Work out the finished part from the listing and answer in its coordinate system (mm). A direction names the side the tool comes from. Give positions to 0.01 mm unless a question says otherwise; leave off trailing zeros. Order: outer loops, then holes, each group sorted by start corner. A loop starts at its lowest first (then second) coordinate and runs counter-clockwise, first axis right, second up. Notation, with made-up numbers: (-5, 43.5) - (28, 43.5) arc R21 ccw to (28, 71.5) - close; hole circle Ø9 at (-34, 18.5). An arc over 180 degrees is marked (long way). Put each result on its own line as item: value.
Autodesk Inventor part; units mm, degrees
ref_plane "YZ Plane" through (0, 0, 0) normal (1, 0, 0) x (0, 1, 0)
ref_plane "XZ Plane" through (0, 0, 0) normal (0, 1, 0) x (-1, 0, 0)
ref_plane "XY Plane" through (0, 0, 0) normal (0, 0, 1) x (1, 0, 0)
sketch "Sketch1" plane through (0, 0, 0) normal (0, 0, 1) x (1, 0, 0)
  line L0 (0, 0) -> (0, 70) construction
  circle A0 centre (0, 0) radius 2.5
  circle A1 centre (0, 70) radius 2.5
  line L1 (0, 0) -> (125, 0) construction
  circle A2 centre (125, 0) radius 2.5
  circle A3 centre (125, 70) radius 2.5
  line L2 (-8.5, -16) -> (133.5, -16)
  line L3 (133.5, -16) -> (133.5, 86)
  line L4 (133.5, 86) -> (-8.5, 86)
  line L5 (-8.5, 86) -> (-8.5, -16)
  point P0 (62.5, 0)
  point P1 (62.5, -16)
  point P2 (0, 35)
  point P3 (-8.5, 35)
  dimension "d0" = 70
  dimension "d1" = 5
  dimension "d2" = 5
  dimension "d3" = 5
  dimension "d4" = 5
  dimension "d5" = 125
  dimension "d6" = 142
  dimension "d7" = 102
extrude "Extrusion1" add sketch "Sketch1" along normal blind 5
sketch "Sketch2" plane through (0, 0, 5) normal (0, 0, 1) x (1, 0, 0)
  line L0 (6.5, 60) -> (118.5, 60)
  line L1 (118.5, 60) -> (118.5, 10)
  line L2 (118.5, 10) -> (6.5, 10)
  line L3 (6.5, 10) -> (6.5, 60)
  line L4 (-8.5, 86) -> (-8.5, -16)
  line L5 (133.5, 86) -> (-8.5, 86)
  point P0 (0, 0)
  point P1 (62.5, 60)
  point P2 (62.5, 86)
  point P3 (6.5, 35)
  point P4 (-8.5, 35)
  dimension "d10" = 15
  dimension "d11" = 50
extrude "Extrusion2" cut sketch "Sketch2" against normal through all
sketch "Sketch3" plane through (-8.5, 86, 0) normal (0, 1, 0) x (1, 0, 0)
  line L0 (142, 0) -> (142, -5)
  line L1 (142, -5) -> (0, -5)
  line L2 (0, -5) -> (0, 80)
  line L3 (0, 80) -> (142, 80)
  line L4 (142, 80) -> (142, -5)
  point P0 (8.5, 0)
  dimension "d17" = 85
extrude "Extrusion3" add sketch "Sketch3" along normal blind 2
sketch "Sketch4" plane through (-8.5, -16, 0) normal (0, -1, 0) x (1, 0, 0)
  line L0 (142, 0) -> (0, 0)
  line L1 (0, 0) -> (0, -80)
  line L2 (0, -80) -> (142, -80)
  line L3 (142, -80) -> (142, 0)
  line L4 (0, 0) -> (142, 0)
  line L5 (142, 0) -> (142, 5)
  line L6 (0, 5) -> (142, 5)
  line L7 (0, 0) -> (0, 5)
  point P0 (8.5, 0)
extrude "Extrusion4" add sketch "Sketch4" along normal blind 2
sketch "Sketch5" plane through (-8.5, 86, -80) normal (-1, 0, 0) x (0, 0, 1)
  line L0 (85, -104) -> (85, 2)
  line L1 (0, -102) -> (0, -104)
  line L2 (85, 2) -> (0, 2)
  line L3 (0, 2) -> (0, -104)
  line L4 (0, -104) -> (85, -104)
  line L5 (85, -104) -> (85, 2)
  point P0 (80, -86)
extrude "Extrusion5" add sketch "Sketch5" along normal blind 2
sketch "Sketch6" plane through (133.5, 86, 0) normal (1, 0, 0) x (0, 0, -1)
  line L0 (-5, -104) -> (-5, 2)
  line L1 (-5, -104) -> (80, -104)
  line L2 (80, -104) -> (80, 2)
  line L3 (80, 2) -> (-5, 2)
  line L4 (-5, 2) -> (-5, -104)
  point P0 (0, -86)
extrude "Extrusion6" add sketch "Sketch6" along normal blind 2
sketch "Sketch7" plane through (0, 0, 5) normal (0, 0, 1) x (1, 0, 0)
  line L0 (118.5, 10) -> (6.5, 10) construction
  line L1 (6.5, 60) -> (118.5, 60) construction
  line L2 (6.5, 10) -> (6.5, 60) construction
  line L3 (118.5, 60) -> (118.5, 10) construction
  line L4 (6.5, 60) -> (61.5, 60)
  line L5 (61.5, 60) -> (61.5, 50)
  line L6 (61.5, 50) -> (6.5, 50)
  line L7 (6.5, 50) -> (6.5, 60)
  line L8 (118.5, 10) -> (63.5, 10)
  line L9 (63.5, 10) -> (63.5, 20)
  line L10 (63.5, 20) -> (118.5, 20)
  line L11 (118.5, 20) -> (118.5, 10)
  line L12 (118.5, 10) -> (6.5, 10)
  line L13 (6.5, 60) -> (118.5, 60)
  line L14 (6.5, 10) -> (6.5, 60)
  point P0 (0, 0)
  point P1 (62.5, 10)
  point P2 (62.5, 60)
  point P3 (6.5, 35)
  dimension "d26" = 55
  dimension "d27" = 10
  dimension "d28" = 55
  dimension "d29" = 10
extrude "Extrusion7" add sketch "Sketch7" against normal blind 5
chamfer "Chamfer2" distance 3 angle 45 4 edges at (35, 10, 0) (90, 60, 0) (91, 20, 5) (34, 50, 5)
sketch "Sketch8" plane through (135.5, 86, 0) normal (1, 0, 0) x (0, 0, -1)
  line L0 (80, -104) -> (80, 2)
  line L1 (80, -102) -> (80, 0)
  line L2 (80, -51) -> (93.9386, -51)
  line L3 (80, -78.0836) -> (55, -78.0836)
  line L4 (55, -78.0836) -> (55, -58.0836)
  line L5 (55, -58.0836) -> (80, -58.0836)
  line L6 (80, -58.0836) -> (80, -78.0836)
  point P0 (0, -86)
  dimension "d36" = 20
  dimension "d37" = 25
  dimension "d40" = 7.0836
extrude "Extrusion8" cut sketch "Sketch8" against normal blind 10
sketch "Sketch9" plane through (-10.5, 86, -80) normal (-1, 0, 0) x (0, 0, 1)
  line L0 (0, -58.0836) -> (0, 0)
  line L1 (0, -31) -> (25, -31)
  line L2 (25, -31) -> (25, -71)
  line L3 (25, -71) -> (0, -71)
  line L4 (0, -71) -> (0, -31)
  line L5 (0, 2) -> (0, -104)
  line L6 (0, -71) -> (25, -71)
  line L7 (25, -71) -> (25, -31)
  line L8 (25, -31) -> (0, -31)
  line L9 (0, -31) -> (0, -71)
  point P0 (80, -86)
  point P1 (0, -51)
  dimension "d41" = 40
  dimension "d42" = 25
extrude "Extrusion9" cut sketch "Sketch9" against normal blind 10
sketch "Sketch10" plane through (-10.5, 86, -80) normal (-1, 0, 0) x (0, 0, 1)
  circle A0 centre (12.5, -93) radius 1.5
  circle A1 centre (12.5, -9) radius 1.5
  line L0 (12.5, -93) -> (12.5, -9) construction
  line L1 (85, -104) -> (85, 2)
  line L2 (25, -71) -> (0, -71)
  point P0 (80, -86)
  point P1 (85, -51)
  point P2 (12.5, -51)
  point P3 (12.5, -71)
  point P4 (12.5, -71)
  dimension "d45" = 3
  dimension "d46" = 3
  dimension "d47" = 84
extrude "Extrusion10" cut sketch "Sketch10" against normal blind 10
sketch "Sketch11" plane through (0, 0, 5) normal (0, 0, 1) x (1, 0, 0)
  circle A0 centre (0, 0) radius 2.5
  circle A1 centre (0, 70) radius 2.5
  circle A2 centre (125, 0) radius 2.5
  circle A3 centre (125, 70) radius 2.5
extrude "Extrusion11" add sketch "Sketch11" against normal blind 5
sketch "Sketch12" plane through (0, 0, 5) normal (0, 0, 1) x (1, 0, 0)
  line L0 (118.5, 20) -> (118.5, 63)
  line L1 (6.5, 7) -> (118.5, 7)
  line L2 (118.5, 7) -> (118.5, 63)
  line L3 (118.5, 63) -> (6.5, 63)
  line L4 (6.5, 63) -> (6.5, 7)
  point P0 (0, 0)
extrude "Extrusion12" cut sketch "Sketch12" along normal through all both and the other way through all
sketch "Sketch13" plane through (135.5, 86, 0) normal (1, 0, 0) x (0, 0, -1)
  line L0 (55, -58.0836) -> (80, -58.0836)
  line L1 (55, -78.0836) -> (55, -58.0836)
  line L2 (80, -78.0836) -> (55, -78.0836)
  line L3 (80, -58.0836) -> (80, -78.0836)
  line L4 (80, -71) -> (80, -102)
  point P0 (0, -86)
extrude "Extrusion13" add sketch "Sketch13" against normal blind 2
sketch "Sketch15" plane through (135.5, 86, 0) normal (1, 0, 0) x (0, 0, -1)
  line L0 (50, -31) -> (70, -31)
  line L1 (70, -31) -> (70, -16)
  line L2 (70, -16) -> (50, -16)
  line L3 (50, -16) -> (50, -31)
  line L4 (80, -104) -> (80, 2)
  line L5 (80, 2) -> (-5, 2)
  point P0 (0, -86)
  dimension "d64" = 20
  dimension "d65" = 15
  dimension "d66" = 10
  dimension "d67" = 18
extrude "Extrusion15" cut sketch "Sketch15" against normal blind 10
sketch "Sketch16" plane through (135.5, 86, 0) normal (1, 0, 0) x (0, 0, -1)
  line L0 (70, -31) -> (50, -31) construction
  line L1 (50, -16) -> (70, -16) construction
  line L2 (50, -31) -> (50, -16) construction
  line L3 (70, -16) -> (70, -31) construction
  line L4 (70, -31) -> (70, -16) construction
  line L5 (70, -31) -> (38, -31) construction
  line L6 (38, -31) -> (38, -71) construction
  line L7 (38, -71) -> (80, -71) construction
  line L8 (80, -71) -> (80, -31) construction
  line L9 (43, -66) -> (43, -36) construction
  line L10 (43, -36) -> (75, -36) construction
  line L11 (75, -36) -> (75, -66) construction
  line L12 (75, -66) -> (43, -66) construction
  line L13 (43, -36) -> (75, -36)
  line L14 (75, -36) -> (75, -38)
  line L15 (75, -38) -> (43, -38)
  line L16 (43, -38) -> (43, -36)
  line L17 (75, -66) -> (43, -66)
  line L18 (43, -66) -> (43, -64)
  line L19 (43, -64) -> (75, -64)
  line L20 (75, -64) -> (75, -66)
  line L21 (75, -45) -> (43, -45)
  line L22 (43, -43) -> (75, -43) construction
  line L23 (43, -43) -> (75, -43)
  line L24 (75, -43) -> (75, -45)
  line L25 (43, -45) -> (43, -43)
  line L26 (75, -43) -> (75, -73) construction
  line L27 (75, -52) -> (43, -52)
  line L28 (43, -50) -> (75, -50) construction
  line L29 (43, -50) -> (75, -50)
  line L30 (75, -50) -> (75, -52)
  line L31 (43, -52) -> (43, -50)
  line L32 (75, -50) -> (75, -80) construction
  line L33 (75, -59) -> (43, -59)
  line L34 (43, -57) -> (75, -57) construction
  line L35 (43, -57) -> (75, -57)
  line L36 (75, -57) -> (75, -59)
  line L37 (43, -59) -> (43, -57)
  line L38 (75, -57) -> (75, -87) construction
  line L39 (75, -66) -> (43, -66)
  line L40 (43, -64) -> (75, -64) construction
  line L41 (43, -64) -> (75, -64)
  line L42 (75, -64) -> (75, -66)
  line L43 (43, -66) -> (43, -64)
  line L44 (75, -64) -> (75, -94) construction
  line L45 (80, -104) -> (80, 2)
  point P0 (0, -86)
  dimension "d70" = 42
  dimension "d71" = 40
  dimension "d72" = 5
  dimension "d73" = 2
  dimension "d74" = 2
  dimension "d77" = 7
extrude "Extrusion16" cut sketch "Sketch16" against normal blind 10
sketch "Sketch17" plane through (135.5, 86, 0) normal (1, 0, 0) x (0, 0, -1)
  circle A0 centre (67.5, -93) radius 1.5
  point P0 (0, -86)
extrude "Extrusion17" cut sketch "Sketch17" against normal blind 10
properties part number "GA06" material "ABS Plastic"
(1) Section C-C, the plane z = -72.5 is taken. Count the separate pieces of the cut face and the enclosed holes in it, then the cut area to 3 significant figures.
Geometry check:
separate pieces: 6
enclosed holes: 0
area: 892 mm²
(2) Section B-B, the plane x = 85 is taken. Write down the section's boundary in (y, z).
Geometry check:
outline: (-18, -80) - (-16, -80) - (-16, 0) - (7, 0) - (7, 5) - (-18, 5) - close; (63, 0) - (86, 0) - (86, -80) - (88, -80) - (88, 5) - (63, 5) - close
(3) Straight lines are drawn through the part: line 1 (Y direction, x = -9.9, z = -67.5); line 2 (Y direction, x = 17, z = 1.5); line 3 (X direction, y = 34, z = -23.5). For each, find the intervals that lie inside material, in ascending order.
Geometry check:
line 1: y = -18 to -8.5, -5.5 to 15, 55 to 75.5, 78.5 to 88
line 2: y = -18 to 7, 63 to 88
line 3: x = -10.5 to -8.5, 133.5 to 135.5
(4) Section A-A, the plane y = 52 is taken. Write down the section's boundary in (x, z), then the cut area to 3 significant figures.
Geometry check:
outline: (-10.5, -55) - (-8.5, -55) - (-8.5, 0) - (6.5, 0) - (6.5, 5) - (-10.5, 5) - close; (118.5, 0) - (133.5, 0) - (133.5, -80) - (135.5, -80) - (135.5, 5) - (118.5, 5) - close
area: 440 mm²
(5) Determine the mould class of faces 4 (the face through (134.514, -7.575, -68.886)), 5 (the face through (61, 88, -38)), 6 (the face through (61, -1, 5)) for opening direction Y: pulls with the +Y half, pulls with the -Y half, needs draft (parallel to the pull), parting line crosses it, or undercut.
Geometry check:
face 4: undercut
face 5: pulls with the +Y half
face 6: needs draft
(6) Given pin 1 (2.5 mm diameter, centred on y = -7, z = -67.5, fed in from -X); pin 2 (3.5 mm diameter, centred on y = -7, z = -67.5, fed in from +X); pin 3 (5 mm diameter, centred on x = 49, y = 72.5, fed in from -Z), each flat-ended and moving along its own axis, determine where each tip first touches the part or whether it passes through.
Geometry check:
pin 1: passes through
pin 2: stops at x = 135.5
pin 3: stops at z = 0
(7) Section D-D, the plane z = -14.5 is taken. Write down the section's boundary in (x, y).
Geometry check:
outline: (-10.5, -18) - (135.5, -18) - (135.5, 88) - (-10.5, 88) - close; hole (-8.5, -16) - (133.5, -16) - (133.5, 86) - (-8.5, 86) - close
(8) A tool of negligible diameter and unlimited length cuts with its end or side. For faces 1 (the face through (62, 7, 2)), 2 (the face through (62, -16, -39)), 3 (the face through (-9.514, 78.265, -66.694)), from which of +Z, -Z, +X, -X, +Y, -Y can it reach the whole face along a straight path? Write none if from no direction.
Geometry check:
face 1: +Z, -Z
face 2: -Z
face 3: -X
